from build123d import *

# Parameters (mm, degrees)
F0_W     = 20
F0_H     = 20
F1_DEPTH = 12.5


with BuildPart() as f1:
    # F0 (on Front) → F1 (new body, symmetric)
    with BuildSketch(Plane.XZ):
        with Locations((-19.847408, 10)):
            Rectangle(F0_W, F0_H)
        Polygon((-9.847408, 20), (-9.847408, 0), (10.152592, 0), (10.152592, 20), (-0.615767, 20), align=None)
        with BuildLine():
            Line((-29.847408, 40), (-29.847408, 20))
            Line((-29.847408, 20), (-9.847408, 20))
            Line((-9.847408, 20), (-0.615767, 20))
            ThreePointArc((-0.615767, 20), (-12.890606, 26.329441), (-14.852573, 40))
            Line((-14.852573, 40), (-29.847408, 40))
        make_face()
        with Locations((20.152592, 10)):
            Rectangle(F0_W, F0_H)
        with BuildLine():
            Line((-0.615767, 20), (10.152592, 20))
            Line((10.152592, 20), (30.152592, 20))
            Line((30.152592, 20), (30.152592, 40))
            Line((30.152592, 40), (13.621039, 40))
            ThreePointArc((13.621039, 40), (11.659072, 26.329441), (-0.615767, 20))
        make_face()
    extrude(amount=F1_DEPTH, both=True)


solid = f1.part
Here's how the part is built. I have some questions about the finished solid (model axes, mm). Round coordinates to 2 decimals unless told otherwise and drop trailing zeros. Write each loop counter-clockwise with the first axis right and the second up, starting at its lowest first coordinate (ties: lowest second). Pieces come first, ordered by that corner, then holes.
1. Will these pins go through, and if not, where does the flat tip stop? pin 1 Ø2 at (x, y) = (-21.5, -3) entering from -Z; pin 2 Ø10 at (x, y) = (0, -0.5) entering from +Z.
2. Suppose I cut it at C-C (z = 26). List the corners of the cut face in (x, y) for me, and give its area (3 significant figures).
3. Suppose I cut it at B-B (y = -6.5). List the corners of the cut face in (x, z) for me, and give its area (3 significant figures).
4. Suppose I cut it at A-A (z = 37.5). List the corners of the cut face in (x, y) for me, and give its area (3 significant figures).
5. I need wall thicknesses on L1, parallel to X at y = 3.5, z = 34.5; L2, parallel to X at y = -11.25, z = 37; L3, parallel to Z at x = 0.5, y = -7.5. Which ranges of each line are inside material? Lowest first, please.
6. Suppose I cut it at D-D (x = -13). List the corners of the cut face in (y, z) for me.
Answer sheet:
1. pin 1: stops at z = 0
1. pin 2: stops at z = 21.09
2. outline: (-29.85, -12.5) - (-12.65, -12.5) - (-12.65, 12.5) - (-29.85, 12.5) - close; (11.42, -12.5) - (30.15, -12.5) - (30.15, 12.5) - (11.42, 12.5) - close
2. area: 898 mm2
3. outline: (-29.85, 0) - (30.15, 0) - (30.15, 40) - (13.62, 40) arc R15.07 cw to (-0.62, 20) arc R15.07 cw to (-14.85, 40) - (-29.85, 40) - close
3. area: 1,900 mm2
4. outline: (-29.85, -12.5) - (-15.49, -12.5) - (-15.49, 12.5) - (-29.85, 12.5) - close; (14.25, -12.5) - (30.15, -12.5) - (30.15, 12.5) - (14.25, 12.5) - close
4. area: 757 mm2
5. L1: x = -29.85 to -15.67, 14.44 to 30.15
5. L2: x = -29.85 to -15.56, 14.33 to 30.15
5. L3: z = 0 to 20.04
6. outline: (-12.5, 0) - (12.5, 0) - (12.5, 26.49) - (-12.5, 26.49) - close
